from build123d import *

# Parameters (mm, degrees)
SKETCH1_R           = 2.75
BOSS_EXTRUDE1_DEPTH = 3.175


with BuildPart() as part:
    # Sketch1 → Boss-Extrude1 (new body)
    with BuildSketch(Plane.XY):
        Polygon((-122.104796952, -176.121133645), (-122.104796952, -133.399898637), (-181.032796952, -160.878476317), (-181.032796952, -176.121133645), align=None)
        with Locations((-174.682796952, -164.923872473)):
            Circle(SKETCH1_R, mode=Mode.SUBTRACT)
        with Locations((-128.454796952, -143.370341124)):
            Circle(SKETCH1_R, mode=Mode.SUBTRACT)
    extrude(amount=-BOSS_EXTRUDE1_DEPTH)


solid = part.part
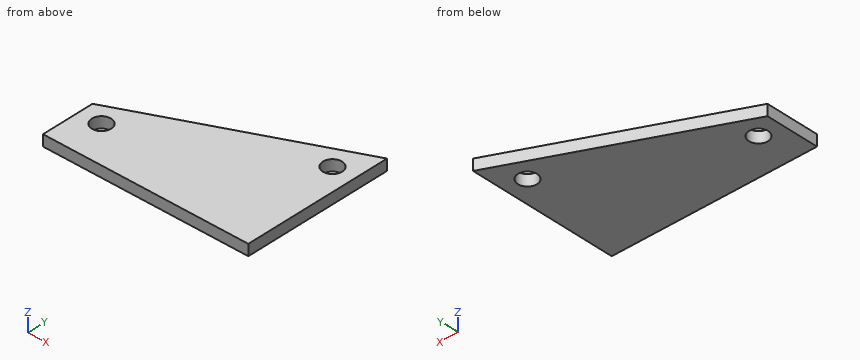
Model file for the job. Use its own axes, mm. Coordinates: 2 decimals unless noted, no trailing zeros. Write each loop counter-clockwise with the first axis right and the second up, starting at its lowest first coordinate (ties: lowest second). Pieces come first, ordered by that corner, then holes. Notation, with made-up numbers: (12.5, -26.75) - (18.5, -26.75) arc R27 ccw to (18.5, 2.25) - close; hole circle Ø10 at (-16.5, 39.5). An arc over 180 degrees is marked (long way). Write each question's results on one line, items separated by ' | '. Start each with the question number.
1) Cut at D-D (y = -139). Write the cut outline in (x, z) (3 decimals).
2) Cut at A-A (y = -163.5). Write the cut outline in (x, z) (3 decimals).
3) Probe line 1 along X through (y, z) = (-163, -1.8); line 2 along X through (y, z) = (-144, -2.5); line 3 along X through (y, z) = (-149.5, -2.35). List the from-to ranges inside material, lowest first. Write a range as from..to.
4) Cut at C-C (z = -2.45). Write the cut outline in (x, y).
5) Cut at B-B (x = -175). Write the cut outline in (y, z) (3 decimals), then the cut area to 3 significant figures.
Returned:
1) outline: (-134.114, -3.175) - (-122.105, -3.175) - (-122.105, 0) - (-134.114, 0) - close
2) outline: (-181.033, -3.175) - (-177.035, -3.175) - (-177.035, 0) - (-181.033, 0) - close; (-172.33, -3.175) - (-122.105, -3.175) - (-122.105, 0) - (-172.33, 0) - close
3) line 1: -181.03..-176.65, -172.72..-122.1 | line 2: -144.84..-131.13, -125.78..-122.1 | line 3: -156.63..-122.1
4) outline: (-181.03, -176.12) - (-122.1, -176.12) - (-122.1, -133.4) - (-181.03, -160.88) - close; hole circle Ø5.5 at (-174.68, -164.92); hole circle Ø5.5 at (-128.45, -143.37)
5) outline: (-176.121, -3.175) - (-167.656, -3.175) - (-167.656, 0) - (-176.121, 0) - close; (-162.192, -3.175) - (-158.065, -3.175) - (-158.065, 0) - (-162.192, 0) - close | area: 40.0 mm^2
